Source: CAD feature listing. Evaluate the final solid. Frame: model axes, mm. Round coordinates to 2 decimals unless told otherwise and drop trailing zeros.
Item 1: First-contact query: P1, Ø4.5, axis at x = 5.5, y = 60.5, coming from the +Z side; P2, Ø1.6, axis at x = 1.74, y = 197.83, coming from the -Z side. Flat tips, straight axial feed; report the tip coordinate or a pass-through.
Item 2: Section query A-A on z = -2.5. Give the number of separate pieces and of enclosed holes in the cut face, then the cut area to 3 significant figures.
Item 3: Pull-direction query (Z, two-part tool) for faces 1 (the flat face through (9.86, 51.167, -3.289)), 2 (the flat face through (10, 200, -2)), 3 (the flat face through (9.86, 7.96, -3.23)), 4 (the flat face through (10, 91, -6)); classes: released by +Z, released by -Z, zero draft, split by the parting line, or undercut.
Item 4: Ray query, L1, parallel to Y at x = 13.25, z = -0.5; L2, parallel to Z at x = 15, y = 176; L3, parallel to Z at x = 18.75, y = 146. Return the intervals inside material, ascending.
```python
from build123d import *

# Parameters (mm, degrees)
SKETCH3_W           = 20
SKETCH3_H           = 6
BOSS_EXTRUDE1_DEPTH = 200
SKETCH7_R           = 1
SKETCH7_R_2         = 1.5
CUT_EXTRUDE1_DEPTH  = 200
CUT_EXTRUDE2_DEPTH  = 20


with BuildPart() as part:
    # Sketch3 → Boss-Extrude1 (new body)
    with BuildSketch(Plane(origin=(0, 0, 0), x_dir=(1, 0, 0), z_dir=(0, 1, 0))):
        with Locations((10, 3)):
            Rectangle(SKETCH3_W, SKETCH3_H)
    extrude(amount=BOSS_EXTRUDE1_DEPTH)

    # Sketch7 → Cut-Extrude1 (cut)
    with BuildSketch(Plane(origin=(0, 0, -6), x_dir=(-1, 0, 0), z_dir=(0, 0, -1))):
        with Locations((-17.73786558, 197.831954878)):
            Circle(SKETCH7_R)
        with Locations((-9.990864499, 189.820422053)):
            Circle(SKETCH7_R_2)
        with Locations((-1.73786558, 181.831954878)):
            Circle(SKETCH7_R)
        with Locations((-17.73786558, 181.831954878)):
            Circle(SKETCH7_R)
        with Locations((-1.73786558, 197.831954878)):
            Circle(SKETCH7_R)
        with Locations((-17.697443934, 1.992082172)):
            Circle(SKETCH7_R)
        with Locations((-13.512620359, 5.194753276)):
            Circle(SKETCH7_R)
        with Locations((-6.48, 5.194753276)):
            Circle(SKETCH7_R)
        with Locations((-2.3, 1.949379891)):
            Circle(SKETCH7_R)
    extrude(amount=-CUT_EXTRUDE1_DEPTH, mode=Mode.SUBTRACT)

    # Sketch8 → Cut-Extrude2 (cut)
    with BuildSketch(Plane.ZY):
        with BuildLine():
            Line((-3.435173621, 200.001787597), (-6.052585671, 200.001787597))
            Line((-6.052585671, 200.001787597), (-6.052585671, 184.116303831))
            ThreePointArc((-6.052585671, 184.116303831), (-4.253368373, 191.978225379), (-3.435173621, 200.001787597))
        make_face()
        Polygon((-5.013852098, 8.990026394), (-1.404702024, 6.906282628), (-1.404702024, 11.073770161), align=None)
        Polygon((-1.409675828, 13.185368824), (-5.018825902, 15.269112591), (-5.018825902, 11.101625057), align=None)
        Polygon((-5.006834199, 17.287599614), (-1.397684125, 15.203855847), (-1.397684125, 19.371343381), align=None)
        Polygon((-1.40265793, 21.482942044), (-5.011808004, 23.566685811), (-5.011808004, 19.399198277), align=None)
        Polygon((-4.848372599, 63.948540489), (-1.239222525, 61.864796722), (-1.239222525, 66.032284256), align=None)
        Polygon((-1.24419633, 68.143882919), (-4.853346404, 70.227626686), (-4.853346404, 66.060139152), align=None)
        Polygon((-5.03782653, 24.96562567), (-1.428676456, 22.881881903), (-1.428676456, 27.049369437), align=None)
        Polygon((-1.433650261, 29.1609681), (-5.042800335, 31.244711867), (-5.042800335, 27.077224333), align=None)
        Polygon((-5.013997563, 32.648394903), (-1.404847489, 30.564651136), (-1.404847489, 34.73213867), align=None)
        Polygon((-1.409821293, 36.843737333), (-5.018971367, 38.927481099), (-5.018971367, 34.759993566), align=None)
        Polygon((-5.031499061, 40.282604028), (-1.422348987, 38.198860261), (-1.422348987, 42.366347795), align=None)
        Polygon((-1.427322791, 44.477946458), (-5.036472865, 46.561690225), (-5.036472865, 42.394202691), align=None)
        Polygon((-5.062933803, 48.028503916), (-1.453783729, 45.944760149), (-1.453783729, 50.112247683), align=None)
        Polygon((-1.458757534, 52.223846346), (-5.067907608, 54.307590112), (-5.067907608, 50.140102579), align=None)
        Polygon((-5.064343036, 55.954978053), (-1.455192962, 53.871234286), (-1.455192962, 58.03872182), align=None)
        Polygon((-1.460166767, 60.150320483), (-5.069316841, 62.23406425), (-5.069316841, 58.066576716), align=None)
        Polygon((-4.841354701, 72.246113708), (-1.232204627, 70.162369942), (-1.232204627, 74.329857475), align=None)
        Polygon((-1.237178431, 76.441456138), (-4.846328505, 78.525199905), (-4.846328505, 74.357712372), align=None)
        Polygon((-4.872347032, 79.924139765), (-1.263196958, 77.840395998), (-1.263196958, 82.007883531), align=None)
        Polygon((-1.268170762, 84.119482194), (-4.877320836, 86.203225961), (-4.877320836, 82.035738428), align=None)
        Polygon((-4.848518064, 87.606908997), (-1.23936799, 85.523165231), (-1.23936799, 89.690652764), align=None)
        Polygon((-1.244341795, 91.802251427), (-4.853491869, 93.885995194), (-4.853491869, 89.71850766), align=None)
        Polygon((-4.866019563, 95.241118123), (-1.256869489, 93.157374356), (-1.256869489, 97.324861889), align=None)
        Polygon((-1.261843293, 99.436460552), (-4.870993367, 101.520204319), (-4.870993367, 97.352716786), align=None)
        Polygon((-4.897454305, 102.98701801), (-1.288304231, 100.903274244), (-1.288304231, 105.070761777), align=None)
        Polygon((-1.293278035, 107.18236044), (-4.902428109, 109.266104207), (-4.902428109, 105.098616674), align=None)
        Polygon((-4.898863538, 110.913492147), (-1.289713464, 108.829748381), (-1.289713464, 112.997235914), align=None)
        Polygon((-1.294687269, 115.108834577), (-4.903837343, 117.192578344), (-4.903837343, 113.025090811), align=None)
        Polygon((-4.725469308, 118.775061554), (-1.116319234, 116.691317787), (-1.116319234, 120.858805321), align=None)
        Polygon((-1.121293038, 122.970403984), (-4.730443112, 125.05414775), (-4.730443112, 120.886660217), align=None)
        Polygon((-4.71845141, 127.072634773), (-1.109301336, 124.988891007), (-1.109301336, 129.15637854), align=None)
        Polygon((-1.11427514, 131.267977203), (-4.723425214, 133.35172097), (-4.723425214, 129.184233436), align=None)
        Polygon((-4.749443741, 134.750660829), (-1.140293667, 132.666917063), (-1.140293667, 136.834404596), align=None)
        Polygon((-1.145267471, 138.946003259), (-4.754417545, 141.029747026), (-4.754417545, 136.862259493), align=None)
        Polygon((-4.725614773, 142.433430062), (-1.116464699, 140.349686295), (-1.116464699, 144.517173829), align=None)
        Polygon((-1.121438503, 146.628772492), (-4.730588577, 148.712516259), (-4.730588577, 144.545028725), align=None)
        Polygon((-4.743116271, 150.067639187), (-1.133966197, 147.983895421), (-1.133966197, 152.151382954), align=None)
        Polygon((-1.138940002, 154.262981617), (-4.748090076, 156.346725384), (-4.748090076, 152.179237851), align=None)
        Polygon((-4.774551014, 157.813539075), (-1.16540094, 155.729795309), (-1.16540094, 159.897282842), align=None)
        Polygon((-1.170374744, 162.008881505), (-4.779524818, 164.092625272), (-4.779524818, 159.925137738), align=None)
        Polygon((-4.775960247, 165.740013212), (-1.166810173, 163.656269446), (-1.166810173, 167.823756979), align=None)
        Polygon((-1.171783977, 169.935355642), (-4.780934051, 172.019099409), (-4.780934051, 167.851611875), align=None)
        Polygon((-4.95123506, 174.038440061), (-1.342084986, 171.954696294), (-1.342084986, 176.122183828), align=None)
        Polygon((-1.34705879, 178.233782491), (-4.956208864, 180.317526258), (-4.956208864, 176.150038724), align=None)
    extrude(amount=-CUT_EXTRUDE2_DEPTH, mode=Mode.SUBTRACT)


solid = part.part
```
Data:
1. P1: stops at z = 0
1. P2: passes through
2. separate pieces: 45
2. enclosed holes: 9
2. area: 2,140 mm2
3. face 1: undercut
3. face 2: zero draft
3. face 3: undercut
3. face 4: released by -Z
4. L1: y = 0 to 4.23, 6.16 to 200
4. L2: z = -6 to -1.55, -1.34 to 0
4. L3: z = -6 to -4.73, -2.21 to 0
